```python
from build123d import *

# Parameters (mm, degrees)
F1_DEPTH = 12.7
F2_T     = -7.62
F3_R     = 5.5188922036
F4_R     = 1.27


with BuildPart() as f1:
    # F0 (on Top) → F1 (new body)
    with BuildSketch(Plane.XY):
        with BuildLine():
            Line((0, -28.8406666368), (0, 0))
            ThreePointArc((0, 0), (-14.4203333184, -14.4203333184), (0, -28.8406666368))
        make_face()
        with BuildLine():
            ThreePointArc((43.2635399552, -14.4203333184), (39.0399221132, -4.223617842), (28.8432066368, 0))
            Line((28.8432066368, 0), (28.8432066368, -28.8406666368))
            ThreePointArc((28.8432066368, -28.8406666368), (39.0399221132, -24.6170487948), (43.2635399552, -14.4203333184))
        make_face()
        with BuildLine():
            Line((28.8432066368, 0), (0, 0))
            ThreePointArc((0, 0), (10.1967154764, -4.223617842), (14.4203333184, -14.4203333184))
            ThreePointArc((14.4203333184, -14.4203333184), (10.1967154764, -24.6170487948), (0, -28.8406666368))
            Line((0, -28.8406666368), (28.8432066368, -28.8406666368))
            ThreePointArc((28.8432066368, -28.8406666368), (14.4228733184, -14.4203333184), (28.8432066368, 0))
        make_face()
        with BuildLine():
            ThreePointArc((14.4203333184, -14.4203333184), (10.1967154764, -4.223617842), (0, 0))
            Line((0, 0), (0, -28.8406666368))
            ThreePointArc((0, -28.8406666368), (10.1967154764, -24.6170487948), (14.4203333184, -14.4203333184))
        make_face()
        with BuildLine():
            Line((28.8432066368, -28.8406666368), (28.8432066368, 0))
            ThreePointArc((28.8432066368, 0), (14.4228733184, -14.4203333184), (28.8432066368, -28.8406666368))
        make_face()
    extrude(amount=F1_DEPTH)

    # F2
    f2_openings = [f1.faces().sort_by_distance(p)[0] for p in [
        (14.421603, -14.420333, 12.7),
        (14.421603, -14.420333, 0),
    ]]
    offset(amount=F2_T, openings=f2_openings)

    # F3
    f3_edges = [f1.edges().sort_by_distance(p)[0] for p in [
        (14.421603, -28.840667, 12.7),
        (14.421603, -28.840667, 0),
    ]]
    fillet(f3_edges, radius=F3_R)

    # F4
    f4_edges = [f1.edges().sort_by_distance(p)[0] for p in [
        (14.421603, -7.62, 0),
        (14.421603, -7.62, 12.7),
    ]]
    fillet(f4_edges, radius=F4_R)


solid = f1.part
```
Could you check a few things on this model? Use its own coordinates, in mm. A direction names the side the tool comes from. Round coordinates to 2 decimals unless told otherwise and drop trailing zeros. Loops run counter-clockwise (first coordinate to the right, second up) from the corner with the lowest first, then second, coordinate; pieces in that order, holes last. Notation, with made-up numbers: (-12.75, 61.25) -> (8.25, 61.25) arc R18 cw to (8.25, 70.25) -> close; hole circle Ø10 at (-39.75, -0.75). An arc over 180 degrees is marked (long way). One line per question, with ' | ' between items.
(1) If I drill on probe 1 along Y at (x, z) = (11, 7.5); probe 2 along Y at (x, z) = (-4, 11.5); probe 3 along X at (y, z) = (-15, 1.5), over which ranges is the centre line in solid material (lowest first)?
Model answer:
probe 1: y = -28.83 to -21.22, -7.62 to -0.01 | probe 2: y = -26.09 to -19.92, -8.92 to -2.75 | probe 3: x = -12.67 to -6.78, 35.62 to 41.51
(2) If we section it at A-A on x = 19: List the corners of the cut face in (y, z) for me, and give its area (3 significant figures).
Model answer:
outline: (-28.84, 5.52) arc R5.52 ccw to (-23.32, 0) -> (-22.49, 0) arc R1.27 ccw to (-21.22, 1.27) -> (-21.22, 11.43) arc R1.27 ccw to (-22.49, 12.7) -> (-23.32, 12.7) arc R5.52 ccw to (-28.84, 7.18) -> close; (-7.62, 1.27) arc R1.27 ccw to (-6.35, 0) -> (-5.52, 0) arc R5.52 ccw to (0, 5.52) -> (0, 7.18) arc R5.52 ccw to (-5.52, 12.7) -> (-6.35, 12.7) arc R1.27 ccw to (-7.62, 11.43) -> close | area: 166 mm^2
(3) For faces 5 (the face through (14.62, -27.27, 1.66)), 6 (the face through (14, -21.221, 6)), 7 (the face through (15, 0, 6)), 8 (the face through (14.624, -21.603, 0.362)), 9 (the face through (14.22, -7.238, 12.338)), which set-ups out of +Z, -Z, +X, -X, +Y, -Y let a thin tool reach every point of the face, with its end or its side?
Model answer:
face 5: -Z, +X, -X, -Y | face 6: +Z, -Z | face 7: +Z, -Z, +X, -X, +Y | face 8: -Z | face 9: +Z
(4) For pin 1 Ø1.5 at (y, z) = (-8, 5) entering from -X; pin 2 Ø6 at (y, z) = (-22, 8) entering from -X; pin 3 Ø5 at (y, z) = (-13, 10.5) entering from -X, each with a flat end and sliding along its axis, tell me the tip position at first contact or that it passes through.
Model answer:
pin 1: stops at x = -13.24 | pin 2: stops at x = -13.65 | pin 3: stops at x = -14.33
(5) Thinking about a two-plate mould opening in X: for faces 1 (the face through (15, -7.62, 6)), 2 (the face through (14.22, -7.238, 0.362)), 3 (the face through (13, -6, 12.7)), 4 (the face through (-14.417, -14.103, 6.338)), which applies, released by +X, released by -X, zero draft, split by the parting line, or undercut?
Model answer:
face 1: undercut | face 2: undercut | face 3: zero draft | face 4: released by -X
(6) If we section it at B-B on z = 9.75: List the corners of the cut face in (x, y) for me, and give its area (3 significant figures).
Model answer:
outline: (0, -28.21) -> (28.84, -28.21) arc R13.79 ccw to (28.84, -0.63) -> (0, -0.63) arc R13.79 ccw to start; hole (0, -21.22) -> (28.84, -21.22) arc R6.8 ccw to (28.84, -7.62) -> (0, -7.62) arc R6.8 ccw to start | area: 855 mm^2
